Print and shaded views of the part. All mm, measured from the part's lowest x, y and z. Round coordinates to 2 decimals unless told otherwise and drop trailing zeros. Write each loop counter-clockwise with the first axis right and the second up, starting at its lowest first coordinate (ties: lowest second). Pieces come first, ordered by that corner, then holes. Notation, with made-up numbers: M -29,71 L 8,71 A20 ccw 8,102 Z; hole C -33,85.5 d5. An arc over 180 degrees is marked long. Write item = value, one per line.
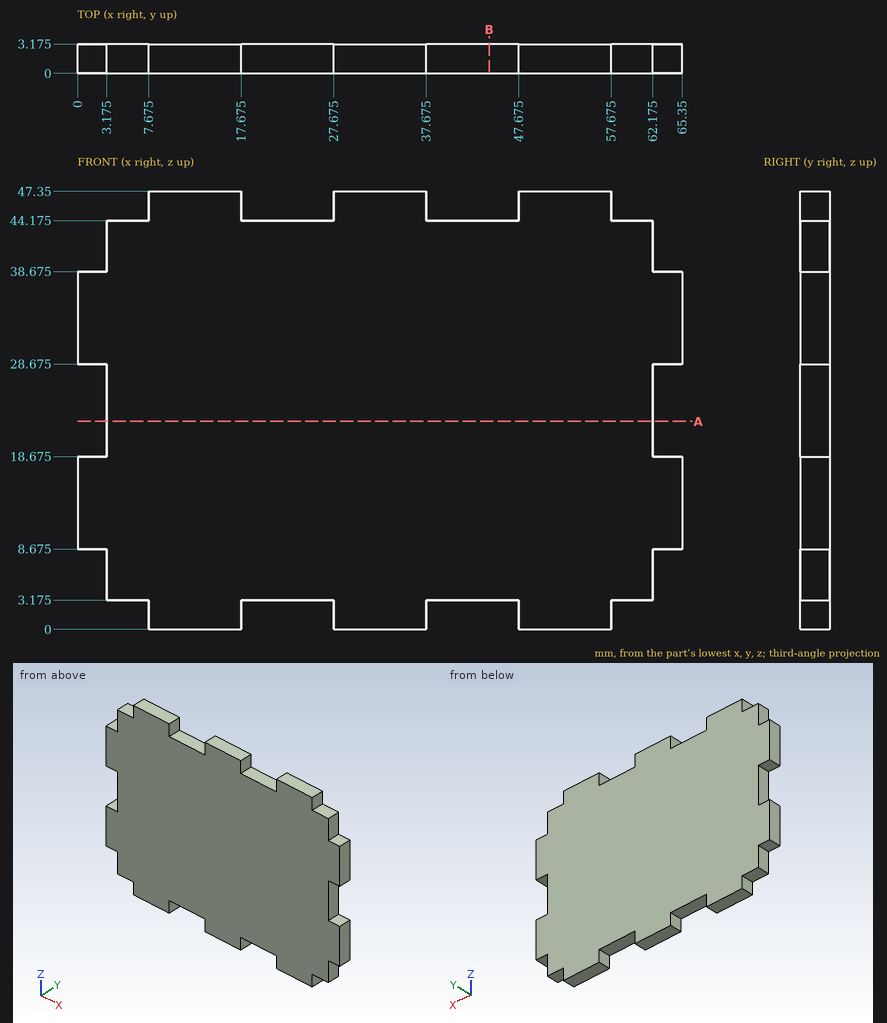
1. Probe probe 1 along X at (y, z) = (3, 2) (3 decimals); probe 2 along Z at (x, y) = (46, 2.5) (3 decimals); probe 3 along X at (y, z) = (2.55, 41) (3 decimals). List the from-to ranges inside material, lowest first.
Responses:
probe_1 = 7.675 to 17.675, 27.675 to 37.675, 47.675 to 57.675
probe_2 = 3.175 to 44.175
probe_3 = 3.175 to 62.175
2. Flat gauge pins, fed straight in: pin 1 (1.6 mm diameter, centred on y = 1.5, z = 46, fed in from +X) (3 decimals); pin 2 (1.6 mm diameter, centred on x = 59.5, y = 1.5, fed in from +Z) (3 decimals); pin 3 (1.6 mm diameter, centred on y = 2, z = 1, fed in from -X) (3 decimals). Where does each tip first touch, or does it go through?
Responses:
pin_1 = 57.675
pin_2 = 44.175
pin_3 = 7.675
3. Band-saw the part on A-A (z = 22.5). List the corners of the cut face in (x, y) (3 decimals).
Responses:
outline = M 3.175,0 L 62.175,0 L 62.175,3.175 L 3.175,3.175 Z
4. Band-saw the part on B-B (x = 44.5). List the corners of the cut face in (y, z) (3 decimals), plus the area to 3 significant figures.
Responses:
outline = M 0,3.175 L 3.175,3.175 L 3.175,44.175 L 0,44.175 Z
area = 130 mm²
